```python
from build123d import *

# Parameters (mm, degrees)
F0_W     = 8.5184480995
F0_H     = 26.1520203203
F0_W_2   = 22.2805645317
F1_DEPTH = 25.4
F2_R     = 21.4623585695
F3_W     = 22.7771224454
F3_H     = 30.0578936003
F4_DEPTH = 3.81


with BuildPart() as f1:
    # F0 (on Top) → F1 (new body)
    with BuildSketch(Plane.XY):
        Polygon((-64.4950717688, 23.875804618), (-64.4950717688, -42.812038213), (8.5184480995, -42.812038213), (8.5184480995, -26.1520203203), (0, -26.1520203203), (0, 0), (8.5184480995, 0), (8.5184480995, 23.875804618), align=None)
        with Locations((4.2592240497, -13.0760101601)):
            Rectangle(F0_W, F0_H)
        with Locations((19.6587303653, -13.0760101601)):
            Rectangle(F0_W_2, F0_H)
    extrude(amount=F1_DEPTH)

    # F2
    f2_edges = [f1.edges().sort_by_distance(p)[0] for p in [
        (-64.495072, -9.468117, 25.4),
    ]]
    fillet(f2_edges, radius=F2_R)

    # F3 (on face) → F4 (join)
    with BuildSketch(Plane.XY.offset(25.4)):
        with Locations((-21.1946009658, -9.6237577964)):
            Rectangle(F3_W, F3_H)
    extrude(amount=-F4_DEPTH)


solid = f1.part
```
The model under review builds one solid part; all positions refer to its coordinate system, in mm. A direction names the side the tool comes from. Round coordinates to 2 decimals unless told otherwise and drop trailing zeros. Loops run counter-clockwise (first coordinate to the right, second up) from the corner with the lowest first, then second, coordinate; pieces in that order, holes last. Notation, with made-up numbers: M 26,52.5 L 57,52.5 A13 ccw 57,77.5 Z; hole C 17,-14 d5. An arc over 180 degrees is marked long. Answer as a JSON object with one key per item and string values.
(1) Take a section at A-A on y = -1. Give the boundary of the cut face in (x, z), and give its area (3 significant figures).
Resolved:
{"outline": "M -64.5,0 L 30.8,0 L 30.8,25.4 L -43.03,25.4 A21.46 ccw -64.5,3.94 Z", "area": "2,320 mm²"}
(2) Take a section at C-C on x = 11. Give the boundary of the cut face in (y, z), and give its area (3 significant figures).
Resolved:
{"outline": "M -26.15,0 L 0,0 L 0,25.4 L -26.15,25.4 Z", "area": "664 mm²"}
(3) Take a section at D-D on y = 16.5. Give the boundary of the cut face in (x, z).
Resolved:
{"outline": "M -64.5,0 L 8.52,0 L 8.52,25.4 L -43.03,25.4 A21.46 ccw -64.5,3.94 Z"}
(4) To check wall thickness, follow line 1 along X through (y, z) = (-39, 2); line 2 along Y through (x, z) = (9.5, 22.5); line 3 along X through (y, z) = (-29.5, 22.5). State the ranges of each line that lie inside material, in increasing order.
Resolved:
{"line 1": "-64.5 to 8.52", "line 2": "-26.15 to 0", "line 3": "-53.81 to 8.52"}
(5) Take a section at B-B on z = 22. Give the boundary of the cut face in (x, y).
Resolved:
{"outline": "M -54.63,-42.81 L 8.52,-42.81 L 8.52,-26.15 L 30.8,-26.15 L 30.8,0 L 8.52,0 L 8.52,23.88 L -54.63,23.88 Z"}
(6) Clearance check with flat-ended pins moving along their axes: P1, Ø6.5, axis at x = 23, z = 9.5, coming from the +Y side; P2, Ø11, axis at x = 20, z = 10, coming from the -Y side; P3, Ø12, axis at y = 8, z = 6.5, coming from the +X side; P4, Ø8, axis at x = 15.5, y = 9, coming from the -Z side. State where each tip first meets the part, or that it passes through.
Resolved:
{"P1": "y = 0", "P2": "y = -26.15", "P3": "x = 8.52", "P4": "through"}
(7) Tool access review of faces 1 (the flat face through (20, 0, 13)), 2 (the flat face through (8.518, -35, 13)), 3 (the cylindrical face through (-58.37, -9.93, 18.95)): name each direction out of +Z, -Z, +X, -X, +Y, -Y from which nothing blocks a thin tool from reaching the whole face with its end or side.
Resolved:
{"face 1": "+Z, -Z, +X, +Y", "face 2": "+Z, -Z, +X, -Y", "face 3": "+Z, -X, +Y, -Y"}
